from build123d import *

# Parameters (mm, degrees)
SKETCH_1_R          = 8
EXTRUDE_1_DEPTH     = 25
SKETCH_2_R          = 12.5
EXTRUDE_2_DEPTH     = 5
SKETCH_3_R          = 1.75
CUT_EXTRUDE_1_DEPTH = 38


with BuildPart() as part:
    # 草图1 → 凸台-拉伸1 (new body)
    with BuildSketch(Plane.XY):
        Circle(SKETCH_1_R)
    extrude(amount=EXTRUDE_1_DEPTH)

    # 草图2 → 凸台-拉伸2 (add)
    with BuildSketch(Plane.XY.offset(25)):
        Circle(SKETCH_2_R)
    extrude(amount=EXTRUDE_2_DEPTH)

    # 草图3 → 切除-拉伸1 (cut)
    with BuildSketch(Plane.XY.offset(30)):
        Circle(SKETCH_3_R)
        with Locations((0, 8)):
            Circle(SKETCH_3_R)
        with Locations((-6.92820323, -4)):
            Circle(SKETCH_3_R)
        with Locations((6.92820323, -4)):
            Circle(SKETCH_3_R)
    extrude(amount=-CUT_EXTRUDE_1_DEPTH, mode=Mode.SUBTRACT)


solid = part.part
Can you work these out from the model? Positions are in its coordinate system, mm. A direction names the side the tool comes from. Give positions to 0.01 mm unless a question says otherwise; leave off trailing zeros. Loops run counter-clockwise (first coordinate to the right, second up) from the corner with the lowest first, then second, coordinate; pieces in that order, holes last. Notation, with made-up numbers: (2.25, -30) - (10.25, -30) arc R24 ccw to (10.25, 4) - close; hole circle Ø6 at (47, 61). An arc over 180 degrees is marked (long way). Return JSON: item names as keys, results as strings.
1. I'm going to push flat-ended pins straight in: pin 1 Ø4 at (x, y) = (-9, -8) entering from -Z; pin 2 Ø6 at (y, z) = (-6.5, 3) entering from +X; pin 3 Ø5 at (x, z) = (8, 12.5) entering from -Y. Where does each tip first touch, or does it pass through?
Output values:
{"pin 1": "stops at z = 25", "pin 2": "stops at x = 5.89", "pin 3": "stops at y = -5.81"}
2. For faces 4 (the face through (0, -3, 30)), 5 (the face through (6.974, 3.919, 12.325)), 6 (the face through (0, -8, 12)), which set-ups out of +Z, -Z, +X, -X, +Y, -Y let a thin tool reach every point of the face, with its end or its side?
Output values:
{"face 4": "+Z, +X, -X, +Y, -Y", "face 5": "-Z, +X", "face 6": "-Z, -Y"}
3. If I drill on line 1 (Y direction, x = 0, z = 9.75); line 2 (X direction, y = -1.5, z = 23.5); line 3 (X direction, y = -9, z = 28.5), over which ranges is the centre line in solid material (lowest first)?
Output values:
{"line 1": "y = -8 to -1.75, 1.75 to 6.25", "line 2": "x = -7.86 to -0.9, 0.9 to 7.86", "line 3": "x = -8.67 to 8.67"}
4. I want a section at B-B on x = -6.75. Please give me the cut outline in (y, z).
Output values:
{"outline": "(-10.52, 25) - (-5.74, 25) - (-5.74, 30) - (-10.52, 30) - close; (-2.26, 0) - (4.29, 0) - (4.29, 25) - (10.52, 25) - (10.52, 30) - (-2.26, 30) - close"}
5. I want a section at A-A on x = 0. Please give me the cut outline in (y, z), and give its area (3 significant figures).
Output values:
{"outline": "(-12.5, 25) - (-8, 25) - (-8, 0) - (-1.75, 0) - (-1.75, 30) - (-12.5, 30) - close; (1.75, 0) - (6.25, 0) - (6.25, 30) - (1.75, 30) - close; (9.75, 25) - (12.5, 25) - (12.5, 30) - (9.75, 30) - close", "area": "359 mm²"}
6. I want a section at C-C on z = 19. Please give me the cut outline in (x, y), and give its area (3 significant figures).
Output values:
{"outline": "(-7.63, -2.4) arc R1.75 cw to (-5.89, -5.41) arc R8 ccw to (5.89, -5.41) arc R1.75 cw to (7.63, -2.4) arc R8 ccw to (1.74, 7.81) arc R1.75 cw to (-1.74, 7.81) arc R8 ccw to start; hole circle Ø3.5 at (0, 0)", "area": "178 mm²"}
7. We'd pull the mould along X, two halves only. Please class faces 1 (the face through (-6.88, 4.08, 12.32)), 2 (the face through (-0.2, -8.2, 25)), 3 (the face through (5.18, -3.92, 18.54)): +X half, -X half, draft (parallel to the pull), parting line (faces both ways), or undercut.
Output values:
{"face 1": "-X half", "face 2": "draft", "face 3": "undercut"}
8. I want a section at D-D on y = -4. Please give me the cut outline in (x, z).
Output values:
{"outline": "(-11.84, 25) - (-8.68, 25) - (-8.68, 30) - (-11.84, 30) - close; (-5.18, 0) - (5.18, 0) - (5.18, 30) - (-5.18, 30) - close; (8.68, 25) - (11.84, 25) - (11.84, 30) - (8.68, 30) - close"}
